Could you check a few things on this drawing? It's one solid part, dimensions in mm from its lowest x, y, z. Coordinates: 2 decimals unless noted, no trailing zeros. Write each loop counter-clockwise with the first axis right and the second up, starting at its lowest first coordinate (ties: lowest second). Pieces come first, ordered by that corner, then holes.
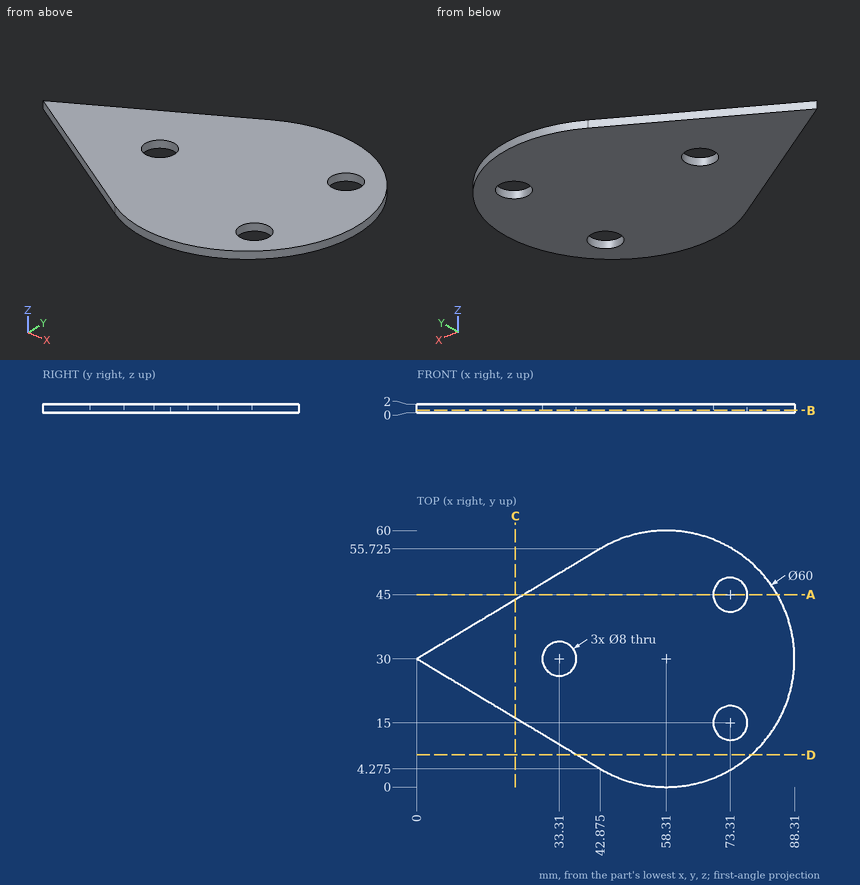
1) Imagine slicing it at C-C on x = 23. Please give me the cut outline in (y, z).
Values follow:
outline: (16.2, 0) - (43.8, 0) - (43.8, 2) - (16.2, 2) - close
2) Imagine slicing it at D-D on y = 7.5. Please give me the cut outline in (x, z).
Values follow:
outline: (37.5, 0) - (78.15, 0) - (78.15, 2) - (37.5, 2) - close
3) Imagine slicing it at A-A on y = 45. Please give me the cut outline in (x, z).
Values follow:
outline: (25, 0) - (69.31, 0) - (69.31, 2) - (25, 2) - close; (77.31, 0) - (84.29, 0) - (84.29, 2) - (77.31, 2) - close
4) Will this pin go through, and if not, where does the flat tip stop? pin 1 (3 mm diameter, centred on x = 51, y = 6, fed in from -Z).
Values follow:
pin 1: stops at z = 0
5) I need wall thicknesses on probe 1 along Y at (x, z) = (74, 0.55); probe 2 along X at (y, z) = (42, 1) (1 decimal); probe 3 along Y at (x, z) = (75, 0.8) (1 decimal). Which ranges of each line are inside material? Lowest first, please.
Values follow:
probe 1: y = 4.43 to 11.06, 18.94 to 41.06, 48.94 to 55.57
probe 2: x = 20 to 70.7, 76 to 85.8
probe 3: y = 5.1 to 11.4, 18.6 to 41.4, 48.6 to 54.9
6) Imagine slicing it at B-B on z = 0.5. Please give me the cut outline in (x, y) (1 decimal), then the cut area to 3 significant figures.
Values follow:
outline: (0, 30) - (42.9, 4.3) arc R30 ccw (long way) to (42.9, 55.7) - close; hole circle Ø8 at (33.3, 30); hole circle Ø8 at (73.3, 15); hole circle Ø8 at (73.3, 45)
area: 3,250 mm2
